Could you check a few things on this drawing? It's one solid part, dimensions in mm from its lowest x, y, z. Coordinates: 2 decimals unless noted, no trailing zeros. Order: outer loops, then holes, each group sorted by start corner. A loop starts at its lowest first (then second) coordinate and runs counter-clockwise, first axis right, second up.
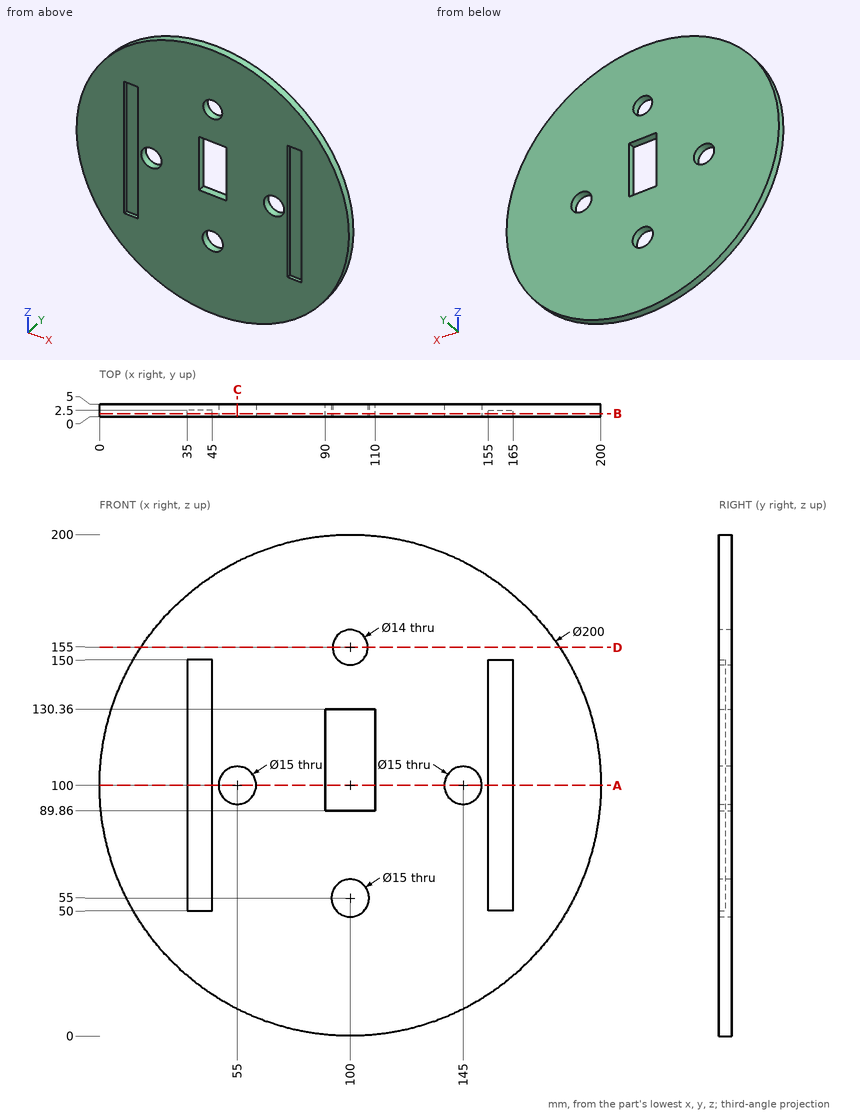
Item 1: Suppose I cut it at B-B (y = 1.2). List the corners of the cut face in (x, z) for me, and give its area (3 significant figures).
Item 2: Suppose I cut it at A-A (z = 100). List the corners of the cut face in (x, y) for me.
Item 3: I need wall thicknesses on line 1 (X direction, y = 2.1, z = 100); line 2 (X direction, y = 1.8, z = 120); line 3 (X direction, y = 4.25, z = 155). Which ranges of each line are inside material? Lowest first, please.
Item 4: Suppose I cut it at C-C (x = 55). List the corners of the cut face in (y, z) for me.
Item 5: Suppose I cut it at D-D (z = 155). List the corners of the cut face in (x, y) for me, and give its area (3 significant figures).
Item 6: For pin 1 Ø0.8 at (y, z) = (1.5, 96.5) entering from -X; pin 2 Ø2 at (x, y) = (177.5, 4.5) entering from -Z; pin 3 Ø0.8 at (y, z) = (1, 77) entering from +X, each with a flat end and sliding along its axis, tell me the tip position at first contact or that it passes through.
Geometry results:
1. outline: circle Ø200 at (100, 100); hole (35, 50) - (45, 50) - (45, 150) - (35, 150) - close; hole circle Ø15 at (55, 100); hole (90, 89.86) - (110, 89.86) - (110, 130.36) - (90, 130.36) - close; hole circle Ø15 at (100, 55); hole circle Ø14 at (100, 155); hole circle Ø15 at (145, 100); hole (155, 50) - (165, 50) - (165, 150) - (155, 150) - close
1. area: 27,900 mm2
2. outline: (0, 0) - (35, 0) - (35, 2.5) - (45, 2.5) - (45, 0) - (47.5, 0) - (47.5, 5) - (0, 5) - close; (62.5, 0) - (90, 0) - (90, 5) - (62.5, 5) - close; (110, 0) - (137.5, 0) - (137.5, 5) - (110, 5) - close; (152.5, 0) - (155, 0) - (155, 2.5) - (165, 2.5) - (165, 0) - (200, 0) - (200, 5) - (152.5, 5) - close
3. line 1: x = 0 to 35, 45 to 47.5, 62.5 to 90, 110 to 137.5, 152.5 to 155, 165 to 200
3. line 2: x = 2.02 to 35, 45 to 90, 110 to 155, 165 to 197.98
3. line 3: x = 16.48 to 93, 107 to 183.52
4. outline: (0, 10.7) - (5, 10.7) - (5, 92.5) - (0, 92.5) - close; (0, 107.5) - (5, 107.5) - (5, 189.3) - (0, 189.3) - close
5. outline: (16.48, 0) - (93, 0) - (93, 5) - (16.48, 5) - close; (107, 0) - (183.52, 0) - (183.52, 5) - (107, 5) - close
5. area: 765 mm2
6. pin 1: stops at x = 0.05
6. pin 2: stops at z = 35.6
6. pin 3: stops at x = 197.41
